```python
from build123d import *

# Parameters (mm, degrees)
BOSS_EXTRUDE1_DEPTH                            = 0.79375
CBORE_FOR_4_BUTTON_HEAD_CAP_SCREW1_D           = 3.2639
CBORE_FOR_4_BUTTON_HEAD_CAP_SCREW1_CBORE_D     = 6.35
CBORE_FOR_4_BUTTON_HEAD_CAP_SCREW1_CBORE_DEPTH = 1.4986
SKETCH6_R                                      = 6.35
BOSS_EXTRUDE2_DEPTH                            = 50.8


with BuildPart() as part:
    # Sketch1 → Boss-Extrude1 (new body)
    with BuildSketch(Plane(origin=(0, 0, 0), x_dir=(1, 0, 0), z_dir=(0, 1, 0))):
        with BuildLine():
            Line((-12.7, -28.575), (-12.7, 28.575))
            ThreePointArc((-12.7, 28.575), (0, 41.275), (12.7, 28.575))
            Line((12.7, 28.575), (12.7, -28.575))
            ThreePointArc((12.7, -28.575), (0, -41.275), (-12.7, -28.575))
        make_face()
    extrude(amount=BOSS_EXTRUDE1_DEPTH)

    # CBORE for #4 Button Head Cap Screw1 (through all)
    with Locations(Plane(origin=(0, 0.79375, 0), x_dir=(-1, 0, 0), z_dir=(0, 1, 0))):
        with Locations((0, 25.4), (0, -25.4)):
            CounterBoreHole(CBORE_FOR_4_BUTTON_HEAD_CAP_SCREW1_D / 2, CBORE_FOR_4_BUTTON_HEAD_CAP_SCREW1_CBORE_D / 2, CBORE_FOR_4_BUTTON_HEAD_CAP_SCREW1_CBORE_DEPTH)

    # Sketch6 → Boss-Extrude2 (add)
    with BuildSketch(Plane(origin=(0, 0.79375, 0), x_dir=(1, 0, 0), z_dir=(0, 1, 0))):
        Circle(SKETCH6_R)
    extrude(amount=BOSS_EXTRUDE2_DEPTH)


solid = part.part
```
The listing builds one solid part. Answer for the finished solid, in the listing's coordinates (mm). A direction names the side the tool comes from. Coordinates: 2 decimals unless noted, no trailing zeros. Loops run counter-clockwise (first coordinate to the right, second up) from the corner with the lowest first, then second, coordinate; pieces in that order, holes last. Notation, with made-up numbers: M 58.25,-20.75 L 81.25,-20.75 A10 cw 81.25,-15.75 Z; hole C -6.75,28 d3. An arc over 180 degrees is marked long. Answer as a JSON object with one key per item and string values. Group by question number.
Item 1: Section B-B (z = 25.4) is taken. Write down the section's boundary in (x, y) (3 decimals), and give its area (3 significant figures).
Item 2: Section D-D (y = 42) is taken. Write down the section's boundary in (x, z), and give its area (3 significant figures).
Item 3: Section C-C (z = 0) is taken. Write down the section's boundary in (x, y).
Item 4: Section A-A (x = 0) is taken. Write down the section's boundary in (y, z) (3 decimals), and give its area (3 significant figures).
Item 5: Determine the mould class of faces 3 (the face through (0.41, 0.4, 28.55)), 4 (the face through (9, 0.794, -1)), 5 (the face through (-0.28, 0.39, -41.27)), 6 (the face through (0.28, 0.39, 41.27)) for opening direction Z: +Z half, -Z half, draft (parallel to the pull), parting line (faces both ways), or undercut.
Item 6: Each of these flat-tipped pins is pushed along its axis until it touches: P1, Ø12, axis at x = 4, y = 20.5, coming from the +Z side; P2, Ø1, axis at x = -2.5, y = 35, coming from the +Z side; P3, Ø3, axis at x = -3, y = 33.5, coming from the -Z side; P4, Ø3, axis at x = 6.5, z = -12.5, coming from the -Y side. Where does it stop, or does it pass through?
Item 7: Consider L1, parallel to Z at x = 0, y = 0.4 (3 decimals); L2, parallel to Z at x = 0.5, y = 34.5; L3, parallel to Y at x = -4.5, z = 6.5. Determine where each line is inside the solid, lowest interval first.
Item 8: Which of the six approach directions +Z, -Z, +X, -X, +Y, -Y give full straight-line access (tool end or side, diameter ignored) to faces 1 (the face through (-1.38, 25.84, 6.2)), 2 (the face through (0, 0, -1))?
Solved:
{
 "1": {"outline": "M -12.7,0 L -3.175,0 L -3.175,0.794 L -12.7,0.794 Z; M 3.175,0 L 12.7,0 L 12.7,0.794 L 3.175,0.794 Z", "area": "15.1 mm2"},
 "2": {"outline": "C 0,0 d12.7", "area": "127 mm2"},
 "3": {"outline": "M -12.7,0 L 12.7,0 L 12.7,0.79 L 6.35,0.79 L 6.35,51.59 L -6.35,51.59 L -6.35,0.79 L -12.7,0.79 Z"},
 "4": {"outline": "M 0,-41.275 L 0.794,-41.275 L 0.794,-28.575 L 0,-28.575 Z; M 0,-22.225 L 0.794,-22.225 L 0.794,-6.35 L 51.594,-6.35 L 51.594,6.35 L 0.794,6.35 L 0.794,22.225 L 0,22.225 Z; M 0,28.575 L 0.794,28.575 L 0.794,41.275 L 0,41.275 Z", "area": "701 mm2"},
 "5": {"face 3": "undercut", "face 4": "draft", "face 5": "-Z half", "face 6": "+Z half"},
 "6": {"P1": "stops at z = 6.35", "P2": "stops at z = 6.03", "P3": "stops at z = -6.17", "P4": "stops at y = 0"},
 "7": {"L1": "z = -41.275 to -28.575, -22.225 to 22.225, 28.575 to 41.275", "L2": "z = -6.33 to 6.33", "L3": "y = 0 to 0.79"},
 "8": {"face 1": "+Y", "face 2": "+Z, -Z, +X, -X, -Y"}
}
